Autodesk Inventor part; units mm, degrees
ref_plane "YZ Plane" through (0, 0, 0) normal (1, 0, 0) x (0, 1, 0)
ref_plane "XZ Plane" through (0, 0, 0) normal (0, 1, 0) x (-1, 0, 0)
ref_plane "XY Plane" through (0, 0, 0) normal (0, 0, 1) x (1, 0, 0)
sketch "Sketch1" plane through (0, 0, 0) normal (0, 1, 0) x (-1, 0, 0)
  line L0 (0, 0) -> (60, 0)
  line L1 (55.02, -23.5) -> (55.02, -51.5)
  line L2 (60, -75) -> (0, -75)
  line L3 (0, -75) -> (0, 0)
  line L4 (55.02, -23.5) -> (72.02, -23.5) construction
  line L5 (72.02, -23.5) -> (72.02, -51.5) construction
  line L6 (72.02, -51.5) -> (55.02, -51.5) construction
  line L7 (55.02, -51.5) -> (55.02, -23.5)
  line L8 (72.02, -51.5) -> (55.02, -51.5)
  line L9 (60, -75) -> (72.02, -75)
  line L10 (72.02, -75) -> (72.02, -51.5)
  line L11 (72.02, -23.5) -> (55.02, -23.5)
  line L12 (60, 0) -> (72.02, 0)
  line L13 (72.02, 0) -> (72.02, -23.5)
  point P0 (55.02, -37.5)
  point P1 (63.52, -51.5)
  point P2 (63.52, -51.5)
  dimension "d2" = 28
  dimension "d25" = 8.5
  dimension "d26" = 60
  dimension "d27" = 12.02
  dimension "d28" = 72.02
  dimension "d36" = 17
  dimension "d37" = 23.5
extrude "Extrusion1" add sketch "Sketch1" along normal blind 11.8
sketch "Sketch2" plane through (-55.02, 0, -23.5) normal (0, 0, -1) x (-1, 0, 0)
  circle A0 centre (10.99, 5.9) radius 2
  line L0 (17, 0) -> (17, 11.8)
  point P0 (-55.02, 0)
  dimension "d6" = 4
  dimension "d7" = 6.01
extrude "Extrusion2" cut sketch "Sketch2" against normal blind 2
sketch "Sketch3" plane through (-72.02, 0, -51.5) normal (0, 0, 1) x (1, 0, 0)
  arc A0 (6.01, 2.5893) -> (6.01, 9.1893) centre (6.01, 5.8893) ccw
  line L0 (6.01, 9.1893) -> (0, 9.1893)
  line L1 (0, 0) -> (0, 11.8)
  line L2 (6.01, 2.5893) -> (0, 2.5893)
  point P0 (72.02, 0)
  dimension "d10" = 6.6
  dimension "d21" = 6.01
  dimension "d22" = 6.01
extrude "Extrusion3" cut sketch "Sketch3" against normal blind 3.65
sketch "Sketch4" plane through (-72.02, 0, -75) normal (-1, 0, 0) x (0, 0, 1)
  line L0 (19.85, 10.7643) -> (17.75, 10.7643)
  line L1 (17.75, 10.7643) -> (17.75, 1.0143)
  line L2 (17.75, 1.0143) -> (19.85, 1.0143)
  line L3 (19.85, 1.0143) -> (19.85, 10.7643)
  line L4 (19.85, 2.5893) -> (19.85, 9.1893)
  point P0 (75, 0)
  point P1 (19.85, 5.8893)
  dimension "d13" = 2.1
  dimension "d14" = 9.75
extrude "Extrusion4" cut sketch "Sketch4" against normal blind 10.925
sketch "Sketch5" plane through (-72.02, 0, 0) normal (0, 0, 1) x (1, 0, 0)
  line L0 (17, 0) -> (17, 11.8)
  line L1 (72.02, 11.8) -> (0, 11.8)
  line L2 (17, 0) -> (72.02, 11.8)
  line L3 (72.02, 11.8) -> (72.02, 0)
  line L4 (72.02, 0) -> (17, 0)
extrude "Extrusion5" cut sketch "Sketch5" against normal blind 88.5 contours L2 L3 L4
sketch "Sketch6" plane through (-72.02, 0, -75) normal (0, 0, -1) x (-1, 0, 0)
  line L0 (-72.02, 11.8) -> (-17, 0)
  line L1 (0, 11.8) -> (-72.02, 11.8)
  line L2 (-72.02, 11.8) -> (0, 11.8)
  line L3 (0, 11.8) -> (0, 0)
  line L4 (-17, 0) -> (-17, 11.8)
  line L5 (0, 0) -> (-17, 0)
  line L6 (-17, 0) -> (-72.02, 11.8)
  point P0 (-72.02, 0)
extrude "Extrusion6" add sketch "Sketch6" along normal blind 10
properties part number "hand_right_1"
The listing builds one solid part. Answer for the finished solid, in the listing's coordinates (mm). A direction names the side the tool comes from. Coordinates: 2 decimals unless noted, no trailing zeros. Loops run counter-clockwise (first coordinate to the right, second up) from the corner with the lowest first, then second, coordinate; pieces in that order, holes last.
1) Find section B-B on y = 5.9. Write down the section's boundary in (x, z) (3 decimals).
2) Find section C-C on z = -28. Write down the section's boundary in (x, y), then the cut area to 3 significant figures.
3) Find the intervals of material crossed by L1, parallel to Y at x = -66, z = -23; L2, parallel to Z at x = -60, y = 0.75; L3, parallel to Y at x = -30.5, z = -30.5, in increasing order.
4) Flat-ended cylindrical pins translate along their axes: pin 1 Ø2 at (x, z) = (-33, -60) entering from -Y; pin 2 Ø3 at (y, z) = (4, -46) entering from -X. Find the tip coordinate at first contact, or state that the pin passes through.
5) A tool of negligible diameter and unlimited length cuts with its end or side. For faces 1 (the face through (-66, 6, -21.5)), 2 (the face through (-62.71, 5.82, -53.3)), 3 (the face through (-62, 6, -51.5)), 4 (the face through (-36, 11.8, -42)), 5 (the face through (-63, 0, -68)), from which of +Z, -Z, +X, -X, +Y, -Y can it reach the whole face along a straight path? Write none if from no direction.
6) Determine the mould class of faces 6 (the face through (-72.02, 6, -68)), 7 (the face through (-67, 6, -57.25)), 8 (the face through (-67, 10.764, -56)), 9 (the face through (-44, 7, -85)) for opening direction Z: pulls with the +Z half, pulls with the -Z half, needs draft (parallel to the pull), parting line crosses it, or undercut.
7) Find section A-A on x = -57. Write down the section's boundary in (y, z).
8) Find section D-D on x = -29.5. Write down the section's boundary in (y, z), then the cut area to 3 significant figures.
Values:
1. outline: (-72.02, -85) - (-27.51, -85) - (-27.51, 0) - (-72.02, 0) - (-72.02, -23.5) - (-68.01, -23.5) - (-68.01, -21.5) - (-64.01, -21.5) - (-64.01, -23.5) - (-55.02, -23.5) - (-55.02, -51.5) - (-62.71, -51.5) - (-62.71, -55.15) - (-61.095, -55.15) - (-61.095, -57.25) - (-72.02, -57.25) - close
2. outline: (-55.02, 0) - (0, 11.8) - (-55.02, 11.8) - close
2. area: 325 mm2
3. L1: y = 0 to 3.9, 7.9 to 11.8
3. L2: z = -85 to -51.5, -23.5 to 0
3. L3: y = 5.26 to 11.8
4. pin 1: stops at y = 4.51
4. pin 2: stops at x = -55.02
5. face 1: none
5. face 2: -X
5. face 3: -X, +Y, -Y
5. face 4: +Z, -Z, +X, -X, +Y
5. face 5: +Z, -Z, +X, -X, -Y
6. face 6: needs draft
6. face 7: undercut
6. face 8: undercut
6. face 9: pulls with the -Z half
7. outline: (0, -85) - (11.8, -85) - (11.8, -51.5) - (0, -51.5) - close; (0, -23.5) - (11.8, -23.5) - (11.8, 0) - (0, 0) - close
8. outline: (5.47, -85) - (11.8, -85) - (11.8, 0) - (5.47, 0) - close
8. area: 538 mm2
